from build123d import *

# Parameters (mm, degrees)
F0_W     = 25.4
F0_H     = 25.4
F1_DEPTH = 25.4
F2_R     = 8.163201
F3_DEPTH = 12.701


with BuildPart() as f1:
    # F0 (on Front) → F1 (new body)
    with BuildSketch(Plane.XZ):
        Rectangle(F0_W, F0_H)
    extrude(amount=F1_DEPTH)

    # F2 (on Top) → F3 (cut, through all)
    with BuildSketch(Plane.XY):
        with Locations((0, -12.994025)):
            Circle(F2_R)
    extrude(amount=F3_DEPTH, mode=Mode.SUBTRACT)


solid = f1.part
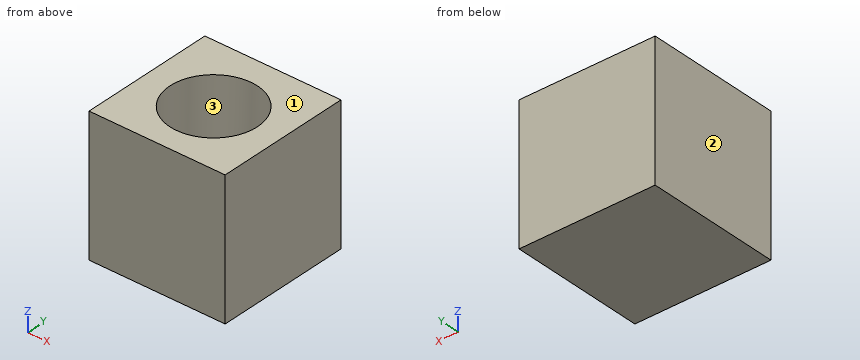
The model under review builds one solid part; all positions refer to its coordinate system, in mm. Face numbers are marked on the shaded views. Round coordinates to 2 decimals unless told otherwise and drop trailing zeros. Loops run counter-clockwise (first coordinate to the right, second up) from the corner with the lowest first, then second, coordinate; pieces in that order, holes last. Notation, with made-up numbers: (63.5, 52.25) -> (114.5, 52.25) arc R29 ccw to (114.5, 86.25) -> close; hole circle Ø3 at (81.5, 73.25). An arc over 180 degrees is marked (long way). Write item = value, one per line. Start each with the question number.
Item 1: Take a section at C-C on y = -7. Give the boundary of the cut face in (x, z), plus the area to 3 significant figures.
Item 2: Mouldability with a two-part tool opening along X and no side actions: class the marked faces 1, 2 and 3 as released by +X, released by -X, zero draft, split by the parting line, or undercut.
Item 3: Take a section at B-B on z = 2.25. Give the boundary of the cut face in (x, y), plus the area to 3 significant figures.
Item 4: Take a section at A-A on x = 0. Give the boundary of the cut face in (y, z), plus the area to 3 significant figures.
Item 5: Insertion check: pin 1 (5 mm diameter, centred on x = 1.5, y = -12, fed in from +Z). The pin has a flat end and moves straight along its axis. Give the tip position at first contact, or say it passes through.
Item 6: To check wall thickness, follow L1, parallel to Y at x = 0, z = 10; L2, parallel to X at y = -6.25, z = 8.25; L3, parallel to X at y = -7.5, z = 10.25. State the ranges of each line that lie inside material, in increasing order.
Result:
q1.outline = (-12.7, -12.7) -> (12.7, -12.7) -> (12.7, 12.7) -> (5.54, 12.7) -> (5.54, 0) -> (-5.54, 0) -> (-5.54, 12.7) -> (-12.7, 12.7) -> close
q1.area = 504 mm²
q2.face_1 = zero draft
q2.face_2 = released by -X
q2.face_3 = undercut
q3.outline = (-12.7, -25.4) -> (12.7, -25.4) -> (12.7, 0) -> (-12.7, 0) -> close; hole circle Ø16.33 at (0, -12.99)
q3.area = 436 mm²
q4.outline = (-25.4, -12.7) -> (0, -12.7) -> (0, 12.7) -> (-4.83, 12.7) -> (-4.83, 0) -> (-21.16, 0) -> (-21.16, 12.7) -> (-25.4, 12.7) -> close
q4.area = 438 mm²
q5.pin_1 = 0
q6.L1 = -25.4 to -21.16, -4.83 to 0
q6.L2 = -12.7 to -4.6, 4.6 to 12.7
q6.L3 = -12.7 to -6.04, 6.04 to 12.7
